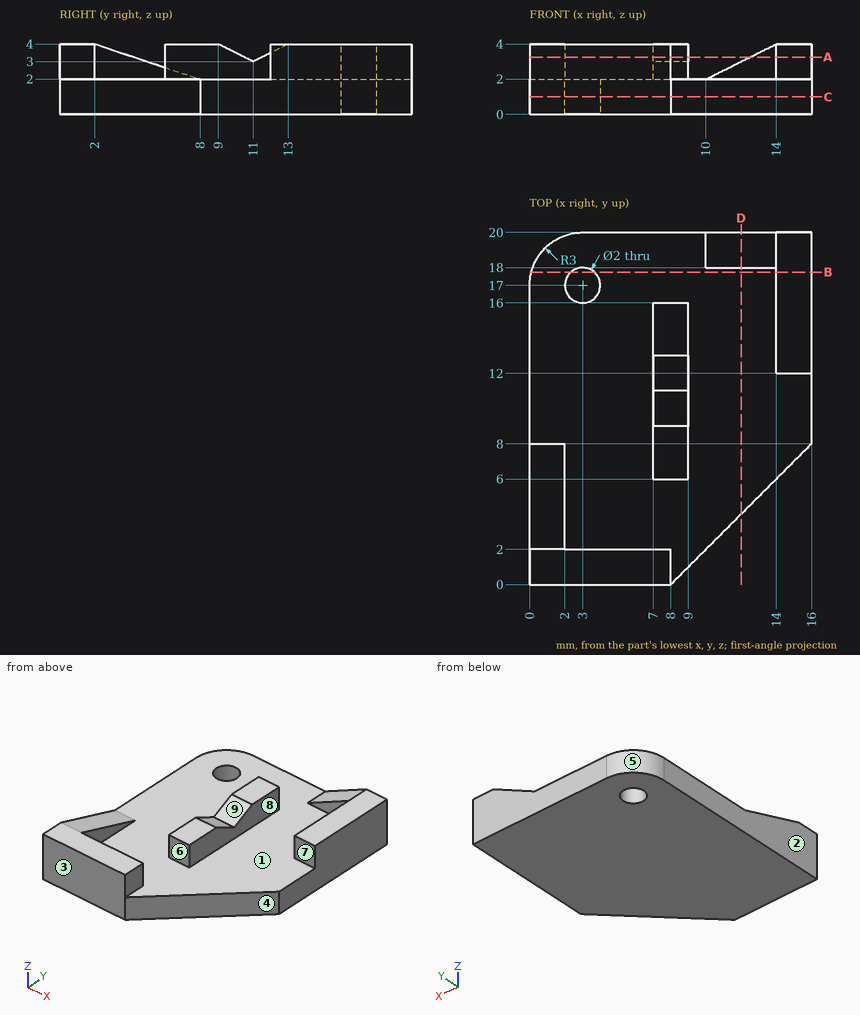
Input: dimensioned drawing with shaded views. Units: mm. Origin: part minimum x, y, z. A direction names the side the tool comes from. Give positions to 0.01 mm unless a question says otherwise; leave off trailing zeros. Loops run counter-clockwise (first coordinate to the right, second up) from the corner with the lowest first, then second, coordinate; pieces in that order, holes last. Notation, with made-up numbers: (85, 34.25) -> (136, 34.25) arc R13 cw to (136, 53.25) -> close; hole circle Ø2 at (72, 73.5). An arc over 180 degrees is marked (long way). Use a Markdown table: item, result. Add a question column.
1) Section query B-B, the plane y = 17.75. Return the cut outline in (x, z).
2) Line query: line 1 along Y through (x, z) = (3, 1.35); line 2 along Y through (x, z) = (7.5, 2.25); line 3 along Y through (x, z) = (12.5, 2.5). Output: solid intervals per line, ascending. Write a range as [from, to].
3) Pull-direction query (X, two-part tool) for the marked faces 1, 2, 3 and 4; classes: +X half, -X half, draft (parallel to the pull), parting line (faces both ways), or undercut.
4) Section query D-D, the plane x = 12. Return the cut outline in (y, z), then the cut area to 3 significant figures.
5) Section query A-A, the plane z = 3.25. Return the cut outline in (x, y), then the cut area to 3 significant figures.
6) First-contact query: pin 1 (0.6 mm diameter, centred on x = 8.5, z = 3, fed in from +Y); pin 2 (1.6 mm diameter, centred on y = 9.5, z = 3, fed in from -X); pin 3 (1.6 mm diameter, centred on y = 4, z = 3, fed in from +X). Flat tips, straight axial feed; report the tip coordinate or a pass-through.
7) Section query C-C, the plane z = 1. Return the cut outline in (x, y), then the cut area to 3 significant figures.
8) Reachability of the marked faces 5, 6, 7, 8 and 9 from +Z, -Z, +X, -X, +Y, -Y: full face, straight path, thin tool, end or side. Return the list, or none.
Numbers:
| question | item | result |
|---|---|---|
| 1 | outline | (0.1, 0) -> (2.34, 0) -> (2.34, 2) -> (0.1, 2) -> close; (3.66, 0) -> (16, 0) -> (16, 4) -> (14, 4) -> (14, 2) -> (3.66, 2) -> close |
| 2 | line 1 | y = [0, 16], [18, 20] |
| 2 | line 2 | y = [0, 2], [6, 16] |
| 2 | line 3 | y = [18, 20] |
| 3 | face 1 | undercut |
| 3 | face 2 | -X half |
| 3 | face 3 | draft |
| 3 | face 4 | +X half |
| 4 | outline | (4, 0) -> (20, 0) -> (20, 3) -> (18, 3) -> (18, 2) -> (4, 2) -> close |
| 4 | area | 34.0 mm2 |
| 5 | outline | (0, 0) -> (8, 0) -> (8, 2) -> (2, 2) -> (2, 4.25) -> (0, 4.25) -> close; (7, 6) -> (9, 6) -> (9, 10.5) -> (7, 10.5) -> close; (7, 11.5) -> (9, 11.5) -> (9, 16) -> (7, 16) -> close; (12.5, 18) -> (14, 18) -> (14, 12) -> (16, 12) -> (16, 20) -> (12.5, 20) -> close |
| 5 | area | 57.5 mm2 |
| 6 | pin 1 | stops at y = 16 |
| 6 | pin 2 | stops at x = 7 |
| 6 | pin 3 | stops at x = 2 |
| 7 | outline | (0, 0) -> (8, 0) -> (16, 8) -> (16, 20) -> (3, 20) arc R3 ccw to (0, 17) -> close; hole circle Ø2 at (3, 17) |
| 7 | area | 283 mm2 |
| 8 | face 5 | +Z, -Z, -X, +Y |
| 8 | face 6 | +Z, +X |
| 8 | face 7 | +Z, +X, -Y |
| 8 | face 8 | +Z, +Y, -Y |
| 8 | face 9 | +Z, -X |
